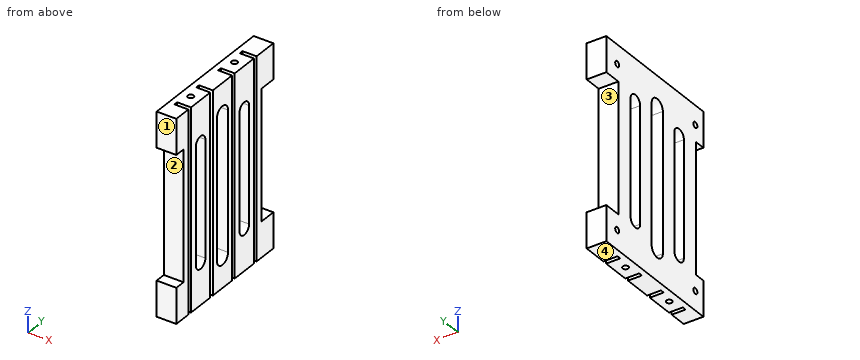
```python
from build123d import *

# Parameters (mm, degrees)
BOSS_EXTRUDE1_DEPTH            = 86.5
M3X0_5_TAPPED_HOLE2_AT_2_COUNT = 2
M3X0_5_TAPPED_HOLE2_AT_2_PITCH = 27.4
M3X0_5_TAPPED_HOLE1_AT_2_COUNT = 2
M3X0_5_TAPPED_HOLE1_AT_2_PITCH = 49
SKETCH14_R                     = 3.5
CUT_EXTRUDE3_DEPTH             = 9.5
CUT_EXTRUDE1_DEPTH             = 9.5
SKETCH15_W                     = 56
SKETCH15_H                     = 7.5
CUT_EXTRUDE4_DEPTH             = 9.5
SKETCH16_W                     = 56
SKETCH16_H                     = 4.5
CUT_EXTRUDE5_DEPTH             = 9.5


with BuildPart() as part:
    # Sketch1 → Boss-Extrude1 (new body)
    with BuildSketch(Plane.XY):
        Polygon((0, 0), (0, 60.8), (8.5, 60.8), (8.5, 50.3), (2.4, 50.3), (2.4, 48.6), (8.5, 48.6), (8.5, 36.6), (2.5, 36.6), (2.5, 34.9), (8.5, 34.9), (8.5, 22.9), (2.5, 22.9), (2.5, 21.2), (8.5, 21.2), (8.5, 9.2), (2.5, 9.2), (2.5, 7.5), (8.5, 7.5), (8.5, 0), align=None)
    extrude(amount=BOSS_EXTRUDE1_DEPTH)

    # Sketch4 → M3x0.5 Tapped Hole2 (revolve, cut)
    with BuildSketch(Plane(origin=(4.25, 42.6, 86.5), x_dir=(0, -1, 0), z_dir=(1, 0, 0))):
        Polygon((0, 0), (0, 6.751075774), (1.25, 6), (1.25, 0), align=None)
    m3x0_5_tapped_hole2 = revolve(axis=Axis((4.25, 42.6, 92.85), (0, 0, -1)), mode=Mode.SUBTRACT)

    # M3x0.5 Tapped Hole2 at 2: M3x0.5 Tapped Hole2 ×2
    with Locations(*[(0, -i * M3X0_5_TAPPED_HOLE2_AT_2_PITCH, 0) for i in range(1, M3X0_5_TAPPED_HOLE2_AT_2_COUNT)]):
        add(m3x0_5_tapped_hole2, mode=Mode.SUBTRACT)

    # Mirror1: M3x0.5 Tapped Hole2 across plane
    add(m3x0_5_tapped_hole2.mirror(Plane.XY.offset(43.25)), mode=Mode.SUBTRACT)

    # Mirror1 copy 1 sketch → Mirror1 copy 1 (revolve, cut)
    with BuildSketch(Plane(origin=(4.25, 15.2, 0), x_dir=(0, -1, 0), z_dir=(1, 0, 0))):
        Polygon((0, 0), (0, -6.751075774), (1.25, -6), (1.25, 0), align=None)
    revolve(axis=Axis((4.25, 15.2, -6.35), (0, 0, -1)), mode=Mode.SUBTRACT)

    # Sketch11 → M3x0.5 Tapped Hole1 (revolve, cut)
    with BuildSketch(Plane(origin=(0, 5, 8.25), x_dir=(0, 0, 1), z_dir=(0, 1, 0))):
        Polygon((0, 0), (0, 4.751075774), (1.25, 4), (1.25, 0), align=None)
    m3x0_5_tapped_hole1 = revolve(axis=Axis((-6.35, 5, 8.25), (1, 0, 0)), mode=Mode.SUBTRACT)

    # M3x0.5 Tapped Hole1 at 2: M3x0.5 Tapped Hole1 ×2
    with Locations(*[(0, i * M3X0_5_TAPPED_HOLE1_AT_2_PITCH, 0) for i in range(1, M3X0_5_TAPPED_HOLE1_AT_2_COUNT)]):
        add(m3x0_5_tapped_hole1, mode=Mode.SUBTRACT)

    # Mirror2: M3x0.5 Tapped Hole1 across plane
    add(m3x0_5_tapped_hole1.mirror(Plane(origin=(0, 0, 43.25), x_dir=(1, 0, 0), z_dir=(0, 0, -1))), mode=Mode.SUBTRACT)

    # Mirror2 copy 1 sketch → Mirror2 copy 1 (revolve, cut)
    with BuildSketch(Plane(origin=(0, 54, 78.25), x_dir=(0, 0, -1), z_dir=(0, 1, 0))):
        Polygon((0, 0), (0, -4.751075774), (1.25, -4), (1.25, 0), align=None)
    revolve(axis=Axis((-6.35, 54, 78.25), (-1, 0, 0)), mode=Mode.SUBTRACT)

    # Sketch14 → Cut-Extrude3 (cut, through all)
    with BuildSketch(Plane(origin=(8.5, 0, 0), x_dir=(0, 0, -1), z_dir=(1, 0, 0))):
        with BuildLine():
            Line((-13.25, 32.4), (-73.25, 32.4))
            ThreePointArc((-73.25, 32.4), (-70.775126266, 31.374873734), (-69.75, 28.9))
            ThreePointArc((-69.75, 28.9), (-70.775126266, 26.425126266), (-73.25, 25.4))
            Line((-73.25, 25.4), (-13.25, 25.4))
            ThreePointArc((-13.25, 25.4), (-16.75, 28.9), (-13.25, 32.4))
        make_face()
        with Locations((-73.25, 28.9)):
            Circle(SKETCH14_R)
        with Locations((-13.25, 28.9)):
            Circle(SKETCH14_R)
    extrude(amount=-CUT_EXTRUDE3_DEPTH, mode=Mode.SUBTRACT)

    # Sketch12 → Cut-Extrude1 (cut, through all)
    with BuildSketch(Plane(origin=(8.5, 0, 0), x_dir=(0, 0, -1), z_dir=(1, 0, 0))):
        with BuildLine():
            Line((-18.25, 45.6), (-68.25, 45.6))
            ThreePointArc((-68.25, 45.6), (-71.25, 42.6), (-68.25, 39.6))
            Line((-68.25, 39.6), (-18.25, 39.6))
            ThreePointArc((-18.25, 39.6), (-15.25, 42.6), (-18.25, 45.6))
        make_face()
        with BuildLine():
            Line((-18.25, 18.2), (-68.25, 18.2))
            ThreePointArc((-68.25, 18.2), (-71.25, 15.2), (-68.25, 12.2))
            Line((-68.25, 12.2), (-18.25, 12.2))
            ThreePointArc((-18.25, 12.2), (-15.25, 15.2), (-18.25, 18.2))
        make_face()
    extrude(amount=-CUT_EXTRUDE1_DEPTH, mode=Mode.SUBTRACT)

    # Sketch15 → Cut-Extrude4 (cut, through all)
    with BuildSketch(Plane(origin=(8.5, 0, 0), x_dir=(0, 0, -1), z_dir=(1, 0, 0))):
        with Locations((-43.25, 57.05)):
            Rectangle(SKETCH15_W, SKETCH15_H)
    extrude(amount=-CUT_EXTRUDE4_DEPTH, mode=Mode.SUBTRACT)

    # Sketch16 → Cut-Extrude5 (cut, through all)
    with BuildSketch(Plane(origin=(8.5, 0, 0), x_dir=(0, 0, -1), z_dir=(1, 0, 0))):
        with Locations((-43.25, 2.25)):
            Rectangle(SKETCH16_W, SKETCH16_H)
    extrude(amount=-CUT_EXTRUDE5_DEPTH, mode=Mode.SUBTRACT)


solid = part.part
```
Can you work these out from the model? Positions are in its coordinate system, mm. Face numbers are marked on the shaded views. Coordinates: 2 decimals unless noted, no trailing zeros. Order: outer loops, then holes, each group sorted by start corner. A loop starts at its lowest first (then second) coordinate and runs counter-clockwise, first axis right, second up.
1. I'm going to push flat-ended pins straight in: pin 1 (2.5 mm diameter, centred on x = 3, z = 53.5, fed in from -Y); pin 2 (3 mm diameter, centred on x = 4.5, z = 63, fed in from +Y); pin 3 (2 mm diameter, centred on x = 4.25, y = 15.2, fed in from +Z). Where does each tip first touch, or does it pass through?
2. If we section it at B-B (z = 32): Give the number of separate pieces and of enclosed holes in the cut face, then the cut area to 3 significant figures.
3. I need wall thicknesses on line 1 (Z direction, x = 2.75, y = 5); line 2 (Z direction, x = 3.75, y = 56); line 3 (X direction, y = 15, z = 4). Which ranges of each line are inside material? Lowest first, please.
4. If we section it at A-A (y = 28.9): Please give me the cut outline in (x, z), then the cut area to 3 significant figures.
5. Thinking about a two-plate mould opening in Z: for the marked faces 1, 2, 3 and 4, which applies, +Z half, -Z half, draft (parallel to the pull), parting line (faces both ways), or undercut?
Entries:
1. pin 1: stops at y = 4.5
1. pin 2: stops at y = 53.3
1. pin 3: stops at z = 80.35
2. separate pieces: 4
2. enclosed holes: 0
2. area: 212 mm2
3. line 1: z = 0 to 7, 9.5 to 77, 79.5 to 86.5
3. line 2: z = 0 to 15.25, 71.25 to 86.5
3. line 3: x = 0 to 3.02, 5.48 to 8.5
4. outline: (0, 0) - (8.5, 0) - (8.5, 9.75) - (0, 9.75) - close; (0, 76.75) - (8.5, 76.75) - (8.5, 86.5) - (0, 86.5) - close
4. area: 166 mm2
5. face 1: draft
5. face 2: undercut
5. face 3: undercut
5. face 4: -Z half
